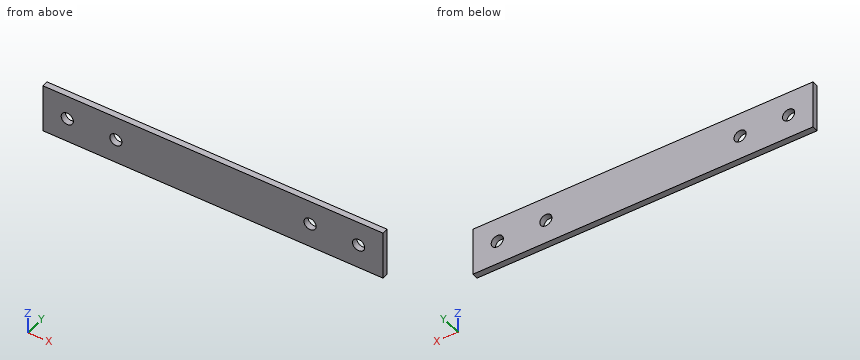
Autodesk Inventor part; units mm, degrees
ref_plane "YZ Plane" through (0, 0, 0) normal (1, 0, 0) x (0, 1, 0)
ref_plane "XZ Plane" through (0, 0, 0) normal (0, 1, 0) x (-1, 0, 0)
ref_plane "XY Plane" through (0, 0, 0) normal (0, 0, 1) x (1, 0, 0)
sketch "Sketch1" plane through (0, 0, 0) normal (1, 0, 0) x (0, 1, 0)
  line L0 (0, 0) -> (3.175, 0)
  line L1 (3.175, 0) -> (3.175, -25.4)
  line L2 (3.175, -25.4) -> (0, -25.4)
  line L3 (0, -25.4) -> (0, 0)
  dimension "d0" = 3.175
  dimension "d1" = 25.4
extrude "Extrusion1" add sketch "Sketch1" along normal blind 177.8
sketch "Sketch2" plane through (0, 3.175, 0) normal (0, 1, 0) x (1, 0, 0)
  line L0 (0, 25.4) -> (0, 0)
  line L1 (0, 12.7) -> (106.9215, 12.7) construction
  circle A0 centre (12.7, 12.7) radius 3.175
  line L2 (0, 25.4) -> (177.8, 25.4)
  line L3 (88.9, 25.4) -> (88.9, 2.1168) construction
  circle A1 centre (38.1, 12.7) radius 3.175
  circle A2 centre (165.1, 12.7) radius 3.175
  circle A3 centre (139.7, 12.7) radius 3.175
  dimension "d4" = 6.35
  dimension "d5" = 50.8
  dimension "d6" = 76.2
extrude "Extrusion2" cut sketch "Sketch2" against normal blind 3.175
properties part number "plate 1"
Input: part model. Units: mm. Frame: model coordinates. Give positions to 0.01 mm unless a question says otherwise; leave off trailing zeros. Order: outer loops, then holes, each group sorted by start corner. A loop starts at its lowest first (then second) coordinate and runs counter-clockwise, first axis right, second up.
Q1. Section C-C on y = 1.3. Output: boundary loops of the cut face in (x, z) (3 decimals), and give its area (3 significant figures).
Checked values:
outline: (0, -25.4) - (177.8, -25.4) - (177.8, 0) - (0, 0) - close; hole circle Ø6.35 at (12.7, -12.7); hole circle Ø6.35 at (38.1, -12.7); hole circle Ø6.35 at (139.7, -12.7); hole circle Ø6.35 at (165.1, -12.7)
area: 4,390 mm2
Q2. Section B-B on z = -12.7. Output: boundary loops of the cut face in (x, y) (3 decimals).
Checked values:
outline: (0, 0) - (9.525, 0) - (9.525, 3.175) - (0, 3.175) - close; (15.875, 0) - (34.925, 0) - (34.925, 3.175) - (15.875, 3.175) - close; (41.275, 0) - (136.525, 0) - (136.525, 3.175) - (41.275, 3.175) - close; (142.875, 0) - (161.925, 0) - (161.925, 3.175) - (142.875, 3.175) - close; (168.275, 0) - (177.8, 0) - (177.8, 3.175) - (168.275, 3.175) - close
Q3. Section A-A on x = 12.7. Output: boundary loops of the cut face in (y, z) (3 decimals), and give its area (3 significant figures).
Checked values:
outline: (0, -25.4) - (3.175, -25.4) - (3.175, -15.875) - (0, -15.875) - close; (0, -9.525) - (3.175, -9.525) - (3.175, 0) - (0, 0) - close
area: 60.5 mm2
Q4. Contact query for flat-ended pins moving along their axis: pin 1 Ø8.5 at (x, z) = (12.7, -12.7) entering from -Y; pin 2 Ø5 at (x, z) = (165.1, -12.7) entering from +Y. Output: stop coordinate, or through.
Checked values:
pin 1: stops at y = 0
pin 2: passes through
Q5. Ray query, probe 1 along X at (y, z) = (1.5, -12.7) (3 decimals); probe 2 along Z at (x, y) = (38.1, 2) (3 decimals); probe 3 along X at (y, z) = (2.5, -11.5). Return the intervals inside material, ascending.
Checked values:
probe 1: x = 0 to 9.525, 15.875 to 34.925, 41.275 to 136.525, 142.875 to 161.925, 168.275 to 177.8
probe 2: z = -25.4 to -15.875, -9.525 to 0
probe 3: x = 0 to 9.76, 15.64 to 35.16, 41.04 to 136.76, 142.64 to 162.16, 168.04 to 177.8
